Source: CAD feature listing. Evaluate the final solid. Frame: model axes, mm. Face numbers are marked on the shaded views. A direction names the side the tool comes from. Round coordinates to 2 decimals unless told otherwise and drop trailing zeros. Write each loop counter-clockwise with the first axis right and the second up, starting at its lowest first coordinate (ties: lowest second). Pieces come first, ordered by that corner, then holes. Notation, with made-up numbers: M 52.25,24 L 84.25,24 A29 cw 84.25,61 Z; hole C 49,28.5 d1. An arc over 180 degrees is marked long. Put each result on its own line as item: value. Start each with the question number.
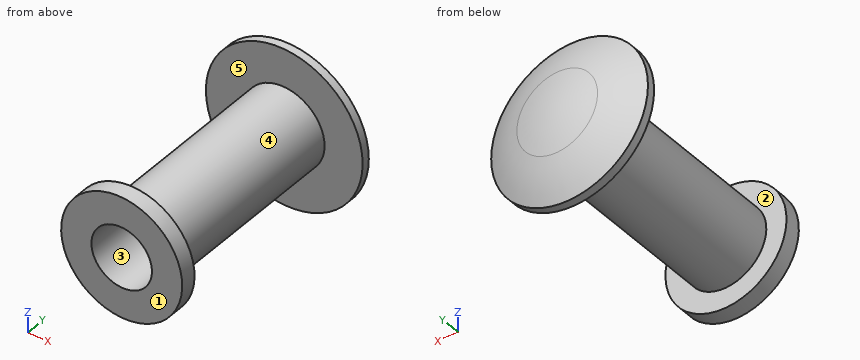
```python
from build123d import *

# Parameters (mm, degrees)
SKETCH_1_W = 4.711910786
SKETCH_1_H = 1


with BuildPart() as part:
    # Эскиз1 → Повернуть1 (revolve)
    with BuildSketch(Plane.XY, mode=Mode.PRIVATE) as revolve_1_sk:
        with BuildLine():
            Line((7.5, 0), (5, 0))
            Line((5, 0), (5, 24.33030278))
            Line((5, 24.33030278), (5, 25.33030278))
            Line((5, 25.33030278), (5, 27.33030278))
            ThreePointArc((5, 27.33030278), (2.522325037, 27.831831467), (0, 28))
            Line((0, 28), (0, 26.5))
            Line((0, 26.5), (2.5, 26.5))
            Line((2.5, 26.5), (2.5, 26))
            Line((2.5, 26), (3.75, 26))
            Line((3.75, 26), (3.75, -2))
            Line((3.75, -2), (7.5, -2))
            Line((7.5, -2), (7.5, 0))
        make_face()
        with BuildLine():
            Line((5, 27.33030278), (5, 25.33030278))
            Line((5, 25.33030278), (9.711910786, 25.33030278))
            ThreePointArc((9.711910786, 25.33030278), (7.423616352, 26.489708981), (5, 27.33030278))
        make_face()
        with Locations((7.355955393, 24.83030278)):
            Rectangle(SKETCH_1_W, SKETCH_1_H)
    revolve(revolve_1_sk.sketch.rotate(Axis((0, -22.043249972, 0), (0, 1, 0)), 90), axis=Axis((0, -22.043249972, 0), (0, 1, 0)))


solid = part.part
```
(1) Ray query, line 1 along X through (y, z) = (11, -0.25); line 2 along X through (y, z) = (26.35, 0); line 3 along Y through (x, z) = (4.25, -5). Return the intervals inside material, ascending.
(2) Section query C-C (x = 0). Return loops of the section in (y, z), and give its area (3 significant figures).
(3) Section query D-D (x = -3). Return loops of the section in (y, z), and give its area (3 significant figures).
(4) Section query B-B (y = 21.25). Return loops of the section in (x, z), and give its area (3 significant figures).
(5) Pull-direction query (Z, two-part tool) for the marked faces 3, 4 and 5; classes: +Z half, -Z half, draft (parallel to the pull), parting line (faces both ways), or undercut.
(6) Contact query for flat-ended pins moving along their axis: P1, Ø4, axis at y = 23.5, z = -5, coming from the -X side; P2, Ø2, axis at y = 18, z = 1.5, coming from the +X side; P3, Ø4, axis at x = 6, y = 11.5, coming from the +Z side; P4, Ø1.5, axis at x = -7, y = 22, coming from the -Z side. Output: stop coordinate, or through.
(7) Section query A-A (z = 0). Return loops of the section in (x, y), and give its area (3 significant figures).
(8) Access query for the marked faces 1 and 2. Directions: +Z, -Z, +X, -X, +Y, -Y. A direction counts if a zero-diameter tool reaches every point of the face in a straight line with its end or side. Return the directions, or none.
Entries:
1. line 1: -4.99 to -3.74, 3.74 to 4.99
1. line 2: -7.74 to -2.5, 2.5 to 7.74
1. line 3: -2 to 0, 24.33 to 26.83
2. outline: M -2,-7.5 L 0,-7.5 L 0,-5 L 24.33,-5 L 24.33,-9.71 L 25.33,-9.71 A19 ccw 25.33,9.71 L 24.33,9.71 L 24.33,5 L 0,5 L 0,7.5 L -2,7.5 L -2,3.75 L 26,3.75 L 26,2.5 L 26.5,2.5 L 26.5,-2.5 L 26,-2.5 L 26,-3.75 L -2,-3.75 Z
2. area: 115 mm2
3. outline: M -2,-6.87 L 0,-6.87 L 0,-4 L 24.33,-4 L 24.33,-9.24 L 25.33,-9.24 A18.76 ccw 25.33,9.24 L 24.33,9.24 L 24.33,4 L 0,4 L 0,6.87 L -2,6.87 L -2,2.25 L 26,2.25 L 26,-2.25 L -2,-2.25 Z
3. area: 145 mm2
4. outline: C 0,0 d10; hole C 0,0 d7.5
4. area: 34.4 mm2
5. face 3: undercut
5. face 4: parting line
5. face 5: draft
6. P1: x = -9.18
6. P2: x = 4.97
6. P3: z = 3
6. P4: through
7. outline: M -9.71,24.33 L -5,24.33 L -5,0 L -7.5,0 L -7.5,-2 L -3.75,-2 L -3.75,26 L -2.5,26 L -2.5,26.5 L 2.5,26.5 L 2.5,26 L 3.75,26 L 3.75,-2 L 7.5,-2 L 7.5,0 L 5,0 L 5,24.33 L 9.71,24.33 L 9.71,25.33 A19 ccw -9.71,25.33 Z
7. area: 115 mm2
8. face 1: +Z, -Z, +X, -X, -Y
8. face 2: none
